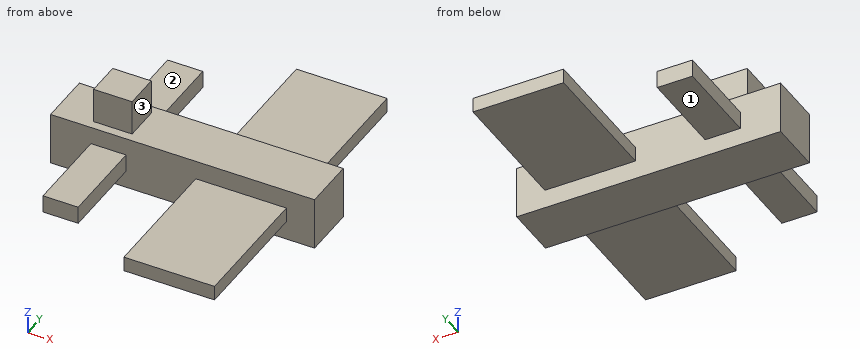
from build123d import *

# Parameters (mm, degrees)
F0_W     = 19.05
F0_H     = 1.905
F1_DEPTH = 3.81
F2_W     = 6.538586
F2_H     = 1.067244
F3_DEPTH = 9.525
F4_W     = 2.54
F4_H     = 1.27
F5_DEPTH = 6.35
F6_W     = 2.782095
F6_H     = 1.268995
F7_DEPTH = 2.54


with BuildPart() as f1:
    # F0 (on Top) → F1 (new body)
    with BuildSketch(Plane.XY):
        with Locations((-56.238926, 5.001349)):
            Rectangle(F0_W, F0_H)
    extrude(amount=F1_DEPTH)

    # F2 (on face) → F3 (join)
    with BuildSketch(Plane(origin=(0, 5.953849, 0), x_dir=(-1, 0, 0), z_dir=(0, 1, 0))):
        with Locations((52.016381, 1.905)):
            Rectangle(F2_W, F2_H)
    extrude(amount=F3_DEPTH)

    # F4 (on face) → F5 (join)
    with BuildSketch(Plane(origin=(0, 5.953849, 0), x_dir=(-1, 0, 0), z_dir=(0, 1, 0))):
        with Locations((61.58399, 1.905)):
            Rectangle(F4_W, F4_H)
    extrude(amount=F5_DEPTH)

    # F6 (on face) → F7 (join)
    with BuildSketch(Plane.XY.offset(3.81)):
        with Locations((-61.618646, 4.683346)):
            Rectangle(F6_W, F6_H)
    extrude(amount=F7_DEPTH)

    # F8: F1 across face


with BuildPart() as f1_1:
    add(f1.part)
    add(f1.part.mirror(Plane(origin=(-56.716231, 4.048849, 2.186695), x_dir=(1, 0, 0), z_dir=(0, -1, 0))))


solid = f1_1.part
Can you work these out from the model? Positions are in its coordinate system, mm. Face numbers are marked on the shaded views. A direction names the side the tool comes from. Coordinates: 2 decimals unless noted, no trailing zeros. Write each loop counter-clockwise with the first axis right and the second up, starting at its lowest first coordinate (ties: lowest second). Pieces come first, ordered by that corner, then holes.
Q1. For P1, Ø7, axis at x = -50.5, y = 12, coming from the -Z side; P2, Ø2, axis at x = -62, z = 4.5, coming from the -Y side; P3, Ø3.5, axis at x = -51.5, y = -0.5, coming from the +Z side; P4, Ø2, axis at x = -57, y = 9, coming from the +Z side, each with a flat end and sliding along its axis, tell me the tip position at first contact or that it passes through.
Results found:
P1: stops at z = 1.37
P2: stops at y = 2.14
P3: stops at z = 2.44
P4: passes through
Q2. Imagine slicing it at D-D, the plane y = 14.25. List the corners of the cut face in (x, z) for me, plus the area to 3 significant figures.
Results found:
outline: (-55.29, 1.37) - (-48.75, 1.37) - (-48.75, 2.44) - (-55.29, 2.44) - close
area: 6.98 mm2
Q3. Please list where these lines run through material, in increasing order: L1, parallel to Z at x = -52, y = -1.75; L2, parallel to Y at x = -60, z = 3; L3, parallel to Y at x = -61.25, z = 5.25.
Results found:
L1: z = 1.37 to 2.44
L2: y = 2.14 to 5.95
L3: y = 2.78 to 5.32
Q4. Imagine slicing it at C-C, the plane z = 2. List the corners of the cut face in (x, y) for me, plus the area to 3 significant figures.
Results found:
outline: (-65.76, 2.14) - (-62.85, 2.14) - (-62.85, -4.21) - (-60.31, -4.21) - (-60.31, 2.14) - (-55.29, 2.14) - (-55.29, -7.38) - (-48.75, -7.38) - (-48.75, 2.14) - (-46.71, 2.14) - (-46.71, 5.95) - (-48.75, 5.95) - (-48.75, 15.48) - (-55.29, 15.48) - (-55.29, 5.95) - (-60.31, 5.95) - (-60.31, 12.3) - (-62.85, 12.3) - (-62.85, 5.95) - (-65.76, 5.95) - close
area: 229 mm2
Q5. Imagine slicing it at A-A, the plane y = 9.5. List the corners of the cut face in (x, z) for me.
Results found:
outline: (-62.85, 1.27) - (-60.31, 1.27) - (-60.31, 2.54) - (-62.85, 2.54) - close; (-55.29, 1.37) - (-48.75, 1.37) - (-48.75, 2.44) - (-55.29, 2.44) - close
Q6. Which directions (+Z, -Z, +X, -X, +Y, -Y) give clear straight access to the entire face, cutting with the end or side of a thin tool? Please do the marked faces 1, 2 and 3.
Results found:
face 1: -Z, +X, -X, +Y
face 2: +Z, +X, -X, +Y
face 3: +Z, +X, +Y, -Y
Q7. Imagine slicing it at B-B, the plane x = -53.5. List the corners of the cut face in (y, z) for me.
Results found:
outline: (-7.38, 1.37) - (2.14, 1.37) - (2.14, 0) - (5.95, 0) - (5.95, 1.37) - (15.48, 1.37) - (15.48, 2.44) - (5.95, 2.44) - (5.95, 3.81) - (2.14, 3.81) - (2.14, 2.44) - (-7.38, 2.44) - close
